Part model, mm, in its own coordinate system. Face numbers are marked on the shaded views. A direction names the side the tool comes from. Give positions to 0.01 mm unless a question says otherwise; leave off trailing zeros. Order: outer loops, then holes, each group sorted by start corner. A loop starts at its lowest first (then second) coordinate and runs counter-clockwise, first axis right, second up. Notation, with made-up numbers: M 36,-13.75 L 94,-13.75 A10 cw 94,-5.75 Z; hole C -30,1.5 d4. An arc over 180 degrees is marked long. Return JSON: item names as keys, results as strings.
Autodesk Inventor part; units mm, degrees
ref_plane "YZ Plane" through (0, 0, 0) normal (1, 0, 0) x (0, 1, 0)
ref_plane "XZ Plane" through (0, 0, 0) normal (0, 1, 0) x (-1, 0, 0)
ref_plane "XY Plane" through (0, 0, 0) normal (0, 0, 1) x (1, 0, 0)
sketch "Boceto1" plane through (0, 0, 0) normal (1, 0, 0) x (0, 1, 0)
  line L0 (27, 0) -> (0, 0)
  line L1 (0, 0) -> (0, 6.55)
  line L2 (0, 6.55) -> (27, 6.55)
  line L3 (27, 6.55) -> (27, 0)
  line L4 (0, 6.55) -> (5, 6.55)
  line L5 (5, 6.55) -> (5, 21.55)
  line L6 (5, 21.55) -> (0, 21.55)
  line L7 (0, 21.55) -> (0, 6.55)
  dimension "d0" = 27
  dimension "d1" = 6.55
  dimension "d2" = 15
  dimension "d3" = 5
extrude "Extrusión1" add sketch "Boceto1" along normal mid plane 17.8
sketch "Boceto4" plane through (-8.9, 5, 21.55) normal (0, 1, 0) x (1, 0, 0)
  point P0 (8.9, 21.55)
sketch "Boceto5" plane through (-8.9, 27, 6.55) normal (0, 1, 0) x (1, 0, 0)
  circle A0 centre (3.8, 3.1) radius 2
  circle A1 centre (14, 3.1) radius 2
  line L0 (0, 0) -> (17.8, 0)
  line L1 (0, 0) -> (0, 6.55)
  line L2 (17.8, 6.55) -> (17.8, 0)
  point P0 (8.9, 6.55)
  dimension "d10" = 4
  dimension "d11" = 4
  dimension "d12" = 3.1
  dimension "d13" = 3.8
  dimension "d14" = 3.8
extrude "Extrusión3" cut sketch "Boceto5" against normal blind 10
sketch "Boceto6" plane through (-8.9, 5, 21.55) normal (0, 1, 0) x (1, 0, 0)
  circle A0 centre (8.9, 7.5) radius 1.75
  line L0 (0, 0) -> (0, 15)
  line L1 (0, 0) -> (17.8, 0)
  point P0 (8.9, 21.55)
  point P1 (0, 7.5)
  point P2 (8.9, 0)
  dimension "d17" = 3.5
extrude "Extrusión4" cut sketch "Boceto6" against normal blind 10
fillet "Empalme1" radius 2 1 edges at (0, 5, 6.55)
fillet "Empalme2" radius 2 1 edges at (0, 5, 21.55)
move faces "Desplazar1" translate (0, 2, 0) faces at (1.6196, 27, 0.4882)
equation "\"d11\" = d10"
equation "\"d14\" = d13"
properties part number "Sujeción de servo a mesa s-c" material "Plástico PC/ABS"
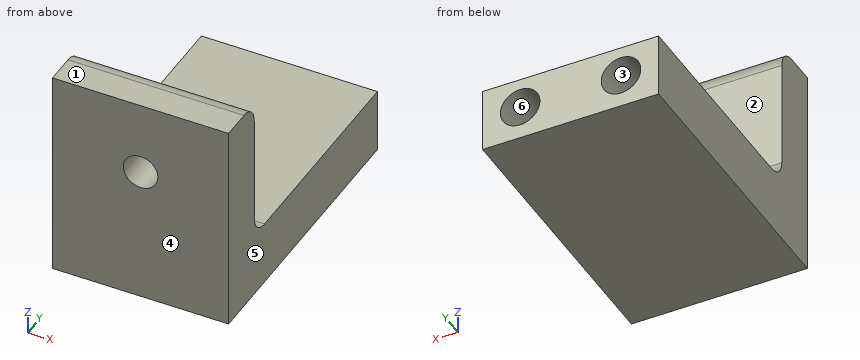
Q1. 3-axis set-ups, long thin cutter, end or side, ignore diameter. For the marked faces 1, 2 and 3: which of +Z, -Z, +X, -X, +Y, -Y reach the whole face in a straight line?
Established:
{"face 1": "+Z, +X, -X, +Y, -Y", "face 2": "+Z, +X, -X, +Y", "face 3": "+Y"}
Q2. Pin check, flat tips, straight feed: pin 1 (3 mm diameter, centred on x = 0, z = 14.05, fed in from +Y); pin 2 (5 mm diameter, centred on x = 6.5, z = 11, fed in from +Y); pin 3 (1.2 mm diameter, centred on x = -5, z = 3.5, fed in from +Y). Stop position of each tip, or through.
Established:
{"pin 1": "passes through", "pin 2": "stops at y = 5", "pin 3": "stops at y = 17"}
Q3. Two-plate mould, pull along X, no slides. Class the marked faces 4, 5 and 6: +X half, -X half, draft (parallel to the pull), parting line (faces both ways), or undercut.
Established:
{"face 4": "draft", "face 5": "+X half", "face 6": "undercut"}
Q4. Band-saw the part on B-B (x = 0). Give the cut face in (y, z).
Established:
{"outline": "M 0,0 L 29,0 L 29,6.55 L 7,6.55 A2 cw 5,8.55 L 5,12.3 L 0,12.3 Z; M 0,15.8 L 5,15.8 L 5,19.55 A2 ccw 3,21.55 L 0,21.55 Z"}
Q5. Probe line 1 along X through (y, z) = (20, 3.45); line 2 along Z through (x, y) = (-5.1, 25.5); line 3 along Z through (x, y) = (0, 1.6). List the from-to ranges inside material, lowest first.
Established:
{"line 1": "x = -8.9 to -7.1, -3.1 to 3.1, 7.1 to 8.9", "line 2": "z = 0 to 1.45, 5.45 to 6.55", "line 3": "z = 0 to 12.3, 15.8 to 21.55"}
Q6. Band-saw the part on D-D (x = -3.5). Give the cut face in (y, z).
Established:
{"outline": "M 0,0 L 29,0 L 29,2.25 L 17,2.25 L 17,4.65 L 29,4.65 L 29,6.55 L 7,6.55 A2 cw 5,8.55 L 5,19.55 A2 ccw 3,21.55 L 0,21.55 Z"}
Q7. Band-saw the part on C-C (z = 3.45). Give the cut face in (x, y).
Established:
{"outline": "M -8.9,0 L 8.9,0 L 8.9,29 L 7.1,29 L 7.1,17 L 3.1,17 L 3.1,29 L -3.1,29 L -3.1,17 L -7.1,17 L -7.1,29 L -8.9,29 Z"}
Q8. Band-saw the part on A-A (z = 14.05). Give the cut face in (x, y), then the cut area to 3 significant figures.
Established:
{"outline": "M -8.9,0 L -1.75,0 L -1.75,5 L -8.9,5 Z; M 1.75,0 L 8.9,0 L 8.9,5 L 1.75,5 Z", "area": "71.5 mm²"}
